Autodesk Inventor part; units mm, degrees
ref_plane "Work Plane1" through (29, 0, 0) normal (0, -1, 0) x (1, 0, 0)
ref_plane "YZ Plane" through (0, 0, 0) normal (1, 0, 0) x (0, 1, 0)
ref_plane "XZ Plane" through (0, 0, 0) normal (0, 1, 0) x (-1, 0, 0)
sketch "Skizze1" plane through (0, 0, 0) normal (0, 0, 1) x (1, 0, 0)
  line L0 (0.3333, 0) -> (12, 0)
  line L1 (12, 0) -> (12, 3)
  line L2 (12, 3) -> (3, 3)
  line L3 (3, 3) -> (2.3864, 3)
  line L4 (2.3864, 3) -> (0, 3)
  line L5 (0, 3) -> (0, 5)
  line L6 (0, 5) -> (-4, 5)
  line L7 (-4, 5) -> (-4, 2.3094)
  line L8 (-4, 2.3094) -> (-1, 2.3094)
  line L9 (-1, 2.3094) -> (0.3333, 0)
  line L10 (-7.2, 0) -> (15.2, 0)
  line L11 (0, -1) -> (0, 6)
  line L12 (3, 3) -> (0, 3) construction
  dimension "d1" = 9
  dimension "d2" = 0.6136
  dimension "d3" = 4
  dimension "d4" = 3
  dimension "d5" = 60
  dimension "d6" = 6
  dimension "d7" = 6
  dimension "d8" = 4.6188
  dimension "d9" = 10
  dimension "d26" = 12
revolve "Körper" add sketch "Skizze1" angle 360 about axis through (0.3333, 0, 0) along (1, 0, 0) contours L9 L11 L4 L3 L2 L1 L0 | L9 L8 L7 L6 L5 L11
sketch "Skizze2" plane through (-4, 0, 0) normal (-1, 0, 0) x (0, 0, 1)
  circle A0 centre (0, 0) radius 2.3094
  line L0 (0, -7) -> (0, 7)
  line L1 (-7, 0) -> (7, 0)
  line L2 (2.3094, 0) -> (1.1547, -2)
  line L3 (1.1547, -2) -> (-1.1547, -2)
  line L4 (-1.1547, -2) -> (-2.3094, 0)
  line L5 (-2.3094, 0) -> (-1.1547, 2)
  line L6 (-1.1547, 2) -> (1.1547, 2)
  line L7 (1.1547, 2) -> (2.3094, 0)
extrude "Loch" add sketch "Skizze2" against normal up to next contours L7 A0 | A0 L2 | L6 L0 A0 | A0 L0 L3 | L0 L6 A0 | A0 L3 L0 | L4 A0 | A0 L5
fillet "Rundung1" radius 0.6 1 edges at (-4, -5, 0)
thread "Gewinde"
chamfer "Fase1" distance 0.6135 distance2 0.6135 1 edges at (12, -3, 0) measured on face at (12, 0.705, 0.3049)
ref_plane "Work Plane1" through (29, 0, 0) normal (0, -1, 0) x (1, 0, 0)
fillet "Fillet2" radius 0.1 1 edges at (0, -3, 0)
equation "\"d1\" = GEL"
equation "\"d3\" = KOH"
equation "\"d4\" = INTI"
equation "\"d6\" = GD"
equation "\"d7\" = BDM"
equation "\"d8\" = 1.1547 * SW"
equation "\"d9\" = KOD"
equation "\"d26\" = NLG"
equation "\"d30\" = R"
equation "\"d17\" = RR"
equation "\"d13\" = GEL"
equation "\"d15\" = -0.5 * SPD + 0.5 * GD"
equation "\"d16\" = GUL"
equation "\"GD\" = NND"
equation "\"NLG\" = 12"
equation "\"GEL\" = 9"
equation "\"KOD\" = 10"
equation "\"KOH\" = 4"
equation "\"INTI\" = 3"
equation "\"GAL\" = 0.61345 * PTC"
equation "\"GUL\" = 0.61345 * PTC"
equation "\"BDM\" = NND"
equation "\"SW\" = 4"
equation "\"RR\" = 0.6"
equation "\"SPD\" = NND - 1.2269 * PTC"
equation "\"R\" = 0.1"
equation "\"TOA\" = 30deg"
equation "\"GD1\" = THREADDIA - 1.2269 * PTC"
equation "\"THREADDIA\" = 6"
equation "\"FAWI\" = 45deg"
equation "\"ANG\" = 120deg"
equation "\"PTC\" = 1"
equation "\"NND\" = 6"
equation "\"E0\" = 1.155 * SW"
properties part number "DIN 7984 - M6 x 12" material "Stahl, weich"
The listing builds one solid part. Answer for the finished solid, in the listing's coordinates (mm). A direction names the side the tool comes from. Round coordinates to 2 decimals unless told otherwise and drop trailing zeros. Loops run counter-clockwise (first coordinate to the right, second up) from the corner with the lowest first, then second, coordinate; pieces in that order, holes last.
Q1. Which of the six approach directions +Z, -Z, +X, -X, +Y, -Y give full straight-line access (tool end or side, diameter ignored) to faces 4 (the face through (-2.433, -1.014, -1.724)), 5 (the face through (-1.72, -1.08, 4.88))?
Q2. Given pin 1 Ø1.5 at (x, z) = (-1.5, -1) entering from -Y; pin 2 Ø5 at (x, z) = (4.5, 3.5) entering from +Y; pin 3 Ø3 at (x, z) = (10, -1.5) entering from +Y, each flat-ended and moving along its own axis, determine where each tip first touches the part or whether it passes through.
Q3. For a pull along Y with two mould halves and no side action, classify faces 1 (the face through (0, 3.3, 0.1)), 2 (the face through (-2.43, 0.99, -1.74)), 3 (the face through (6, -3, 0)) as released by +Y, released by -Y, zero draft, split by the parting line, or undercut.
Q4. Section A-A, the plane x = 8 is taken. Determine the outline of the cut face in (y, z), then the cut area to 3 significant figures.
Q5. Find the intervals of material crossed by line 1 (X direction, y = 4, z = 1); line 2 (X direction, y = -0.25, z = -1.25); line 3 (Z direction, x = 2.25, y = 2), in increasing order.
Completed:
1. face 4: -X
1. face 5: +X, -X
2. pin 1: stops at y = -4.99
2. pin 2: stops at y = 2.83
2. pin 3: stops at y = 3
3. face 1: zero draft
3. face 2: undercut
3. face 3: split by the parting line
4. outline: circle Ø6 at (0, 0)
4. area: 28.3 mm2
5. line 1: x = -4 to 0
5. line 2: x = -0.4 to 12
5. line 3: z = -2.24 to 2.24
